For this review, take the finished solid that the model builds, in its own axes (mm). A direction names the side the tool comes from. Round coordinates to 2 decimals unless told otherwise and drop trailing zeros. Write each loop counter-clockwise with the first axis right and the second up, starting at its lowest first coordinate (ties: lowest second). Pieces come first, ordered by that corner, then holes. Notation, with made-up numbers: (16.25, 58) - (51.25, 58) arc R20 ccw to (51.25, 77) - close; hole circle Ø8 at (-3.75, -38.75). An arc over 180 degrees is marked (long way). One line per item, written item: value. Start each with the question number.
Q1. Add section C-C on x = -16. Write out the cut boundary in (y, z), and give its area (3 significant figures).
Q2. Clearance check with flat-ended pins moving along their axes: pin 1 Ø2.5 at (x, y) = (6.1, -10.5) entering from +Z; pin 2 Ø4.5 at (x, y) = (0, 1) entering from +Z; pin 3 Ø1.5 at (y, z) = (-1.5, 13) entering from +X; pin 4 Ø1.6 at (x, z) = (6.5, -4) entering from +Y. State where each tip first meets the part, or that it passes through.
Q3. Tool access review of faces 4 (the face through (-9.69, -8.603, -17.26)), 5 (the face through (8, -2, 0)), 6 (the face through (-10.854, 2.251, -4.962)): name each direction out of +Z, -Z, +X, -X, +Y, -Y from which nothing blocks a thin tool from reaching the whole face with its end or side.
Q4. Add section A-A on z = -11. Write out the cut boundary in (x, y).
Q5. For probe 1 along X at (y, z) = (-10.5, -16.2); probe 2 along Z at (x, y) = (7.5, -6.75); probe 3 along Z at (x, y) = (-12, -7.75), list the stretches that pass through material, from the lowest coordinate up.
Q6. Add section D-D on z = -0.5. Write out the cut boundary in (x, y).
Q7. Mouldability with a two-part tool opening along X and no side actions: class faces 1 (the face through (8, -2, 12)), 2 (the face through (0, -2.75, 16)), 3 (the face through (-5, -13, 17)) as +X half, -X half, draft (parallel to the pull), parting line (faces both ways), or undercut.
Q8. Add section B-B on y = -10.5. Give the number of separate pieces and of enclosed holes in the cut face, and give its area (3 significant figures).
```python
from build123d import *

# Parameters (mm, degrees)
BOSS_EXTRUDE1_DEPTH   = 18
CROQUIS2_R            = 1.35
CORTAR_EXTRUIR2_DEPTH = 5
SKETCH3_R             = 2.25
CUT_EXTRUDE1_DEPTH    = 1.5
SKETCH5_W             = 5.2
SKETCH5_H             = 5.7
CUT_EXTRUDE2_DEPTH    = 39.212694226
CUT_EXTRUDE3_START    = -15.7
CUT_EXTRUDE3_DEPTH    = 5.4
CROQUIS1_R            = 1.6
CORTAR_EXTRUIR1_DEPTH = 30.883105595
CUT_EXTRUDE7_DEPTH    = 5
SKETCH7_W             = 24.1
SKETCH7_H             = 19.8
CUT_EXTRUDE4_DEPTH    = 5
FILLET5_R             = 2
CHAFL_N1_SIZE         = 5


with BuildPart() as part:
    # Sketch1 → Boss-Extrude1 (new body)
    with BuildSketch(Plane.XY):
        with BuildLine():
            Line((-20, 5.553828843), (-20, -8))
            Line((-20, -8), (-20, -13))
            Line((-20, -13), (11.1, -13))
            Line((11.1, -13), (11.1, -8))
            Line((11.1, -8), (8, -4.9))
            Line((8, -4.9), (8, 0))
            ThreePointArc((8, 0), (5.656854249, 5.656854249), (0, 8))
            Line((0, 8), (-20, 8))
            Line((-20, 8), (-20, 5.553828843))
        make_face()
    boss_extrude1 = extrude(amount=BOSS_EXTRUDE1_DEPTH)

    # Croquis2 → Cortar-Extruir2 (cut)
    with BuildSketch(Plane.XY.offset(18)):
        with Locations((-10.9, -10.5)):
            Circle(CROQUIS2_R)
        with Locations((6.1, -10.5)):
            Circle(CROQUIS2_R)
    cortar_extruir2 = extrude(amount=-CORTAR_EXTRUIR2_DEPTH, mode=Mode.SUBTRACT)

    # Sketch3 → Cut-Extrude1 (cut)
    with BuildSketch(Plane.XY.offset(18)):
        with Locations((-10.9, -10.5)):
            Circle(SKETCH3_R)
        with Locations((6.1, -10.5)):
            Circle(SKETCH3_R)
    cut_extrude1 = extrude(amount=-CUT_EXTRUDE1_DEPTH, mode=Mode.SUBTRACT)

    # Sketch5 → Cut-Extrude2 (cut, through all)
    with BuildSketch(Plane(origin=(11.1, 0, 0), x_dir=(0, 0, -1), z_dir=(1, 0, 0))):
        with Locations((-12.5, -10.15)):
            Rectangle(SKETCH5_W, SKETCH5_H)
    cut_extrude2 = extrude(amount=-CUT_EXTRUDE2_DEPTH, mode=Mode.SUBTRACT)

    # Sketch6 → Cut-Extrude3 (cut)
    with BuildSketch(Plane.XY.offset(18).offset(CUT_EXTRUDE3_START)):
        with BuildLine():
            Line((-13.413555989, 8), (-8.221909119, -3.660629788))
            ThreePointArc((-8.221909119, -3.660629788), (-4.901751315, -7.548035112), (0, -9))
            Line((0, -9), (14.43375673, -9))
            Line((14.43375673, -9), (6.92820323, 4))
            ThreePointArc((6.92820323, 4), (4, 6.92820323), (0, 8))
            Line((0, 8), (-13.413555989, 8))
        make_face()
    cut_extrude3 = extrude(amount=CUT_EXTRUDE3_DEPTH, mode=Mode.SUBTRACT)

    # Croquis1 → Cortar-Extruir1 (cut, through all)
    with BuildSketch(Plane(origin=(0, 0, 0), x_dir=(-1, 0, 0), z_dir=(0, 0, -1))):
        Circle(CROQUIS1_R)
    cortar_extruir1 = extrude(amount=-CORTAR_EXTRUIR1_DEPTH, mode=Mode.SUBTRACT)

    # Sketch10 → Cut-Extrude7 (cut)
    with BuildSketch(Plane.XY.offset(18)):
        Polygon((3.175426481, 0), (1.58771324, 2.75), (-1.58771324, 2.75), (-3.175426481, 0), (-1.58771324, -2.75), (1.58771324, -2.75), align=None)
    cut_extrude7 = extrude(amount=-CUT_EXTRUDE7_DEPTH, mode=Mode.SUBTRACT)

    # Mirror1: Boss-Extrude1, Cortar-Extruir2, Cut-Extrude1, Cut-Extrude2, Cut-Extrude3, Cortar-Extruir1, Cut-Extrude7 across plane
    add(boss_extrude1.mirror(Plane(origin=(0, 0, 0), x_dir=(1, 0, 0), z_dir=(0, 0, -1))))
    add(cortar_extruir2.mirror(Plane(origin=(0, 0, 0), x_dir=(1, 0, 0), z_dir=(0, 0, -1))), mode=Mode.SUBTRACT)
    add(cut_extrude1.mirror(Plane(origin=(0, 0, 0), x_dir=(1, 0, 0), z_dir=(0, 0, -1))), mode=Mode.SUBTRACT)
    add(cut_extrude2.mirror(Plane(origin=(0, 0, 0), x_dir=(1, 0, 0), z_dir=(0, 0, -1))), mode=Mode.SUBTRACT)
    add(cut_extrude3.mirror(Plane(origin=(0, 0, 0), x_dir=(1, 0, 0), z_dir=(0, 0, -1))), mode=Mode.SUBTRACT)
    add(cortar_extruir1.mirror(Plane(origin=(0, 0, 0), x_dir=(1, 0, 0), z_dir=(0, 0, -1))), mode=Mode.SUBTRACT)
    add(cut_extrude7.mirror(Plane(origin=(0, 0, 0), x_dir=(1, 0, 0), z_dir=(0, 0, -1))), mode=Mode.SUBTRACT)

    # Sketch7 → Cut-Extrude4 (cut)
    with BuildSketch(Plane.XZ.offset(13)):
        with Locations((-7.95, 0)):
            Rectangle(SKETCH7_W, SKETCH7_H)
    extrude(amount=-CUT_EXTRUDE4_DEPTH, mode=Mode.SUBTRACT)

    # Fillet5
    fillet5_edges = [part.edges().sort_by_distance(p)[0] for p in [
        (5.656854249, 5.656854249, 18),
        (-10, 8, 18),
        (-10, 8, -18),
        (5.656854249, 5.656854249, -18),
        (8, -2.45, -18),
        (8, -2.45, 18),
    ]]
    fillet(fillet5_edges, radius=FILLET5_R)

    # Chaflán1
    # the kernel refuses this chamfer: 5 mm, written as the material it takes off along each edge
    with BuildSketch(Plane(origin=(4.1, -13, 22.75841494), x_dir=(0.9996219169112968, -0.027495876610586317, 0), z_dir=(0, 0, -1))) as chafl_n1_piece_1_section:
        Polygon((CHAFL_N1_SIZE * 0.999621916911, -CHAFL_N1_SIZE * 0.0274958766106), (-CHAFL_N1_SIZE * 0.0274958766106, -CHAFL_N1_SIZE * 0.999621916911), (0, 0), align=None)
    chafl_n1_piece_1 = extrude(amount=45.51682988, mode=Mode.PRIVATE)
    chafl_n1_piece_1 = split(chafl_n1_piece_1, bisect_by=Plane(origin=(8.49756634, -12.423659296, -15.1), z_dir=(0, 0, 1)), keep=Keep.TOP, mode=Mode.PRIVATE)
    chafl_n1_piece_1 = split(chafl_n1_piece_1, bisect_by=Plane(origin=(8.49756634, -12.423659296, 15.1), z_dir=(0, 0, -1)), keep=Keep.TOP, mode=Mode.PRIVATE)
    add(chafl_n1_piece_1, mode=Mode.SUBTRACT)


solid = part.part
```
Result set:
1. outline: (-13, -18) - (6, -18) arc R2 ccw to (8, -16) - (8, 16) arc R2 ccw to (6, 18) - (-13, 18) - (-13, 15.1) - (-7.3, 15.1) - (-7.3, 9.9) - (-8, 9.9) - (-8, -9.9) - (-7.3, -9.9) - (-7.3, -15.1) - (-13, -15.1) - close
1. area: 596 mm^2
2. pin 1: stops at z = 9.9
2. pin 2: stops at z = 18
2. pin 3: stops at x = 8
2. pin 4: stops at y = -9
3. face 4: -Z
3. face 5: +Z, -Z, +X, +Y
3. face 6: +X, +Y
4. outline: (-20, -7.3) - (10.4, -7.3) - (8, -4.9) - (8, 0) arc R8 ccw to (0, 8) - (-20, 8) - close; hole circle Ø3.2 at (0, 0)
5. probe 1: x = -20 to -12.25, -9.55 to 4.75, 7.45 to 11.1
5. probe 2: z = -18 to -7.7, -2.3 to 2.3, 7.7 to 18
5. probe 3: z = -18 to -15.1, -9.9 to 9.9, 15.1 to 18
6. outline: (-20, -8) - (4.1, -8) - (9.1, -13) - (11.1, -13) - (11.1, -8) - (8, -4.9) - (8, 0) arc R8 ccw to (0, 8) - (-20, 8) - close; hole circle Ø3.2 at (0, 0)
7. face 1: +X half
7. face 2: undercut
7. face 3: draft
8. separate pieces: 7
8. enclosed holes: 0
8. area: 227 mm^2
